```python
from build123d import *

# Parameters (mm, degrees)
F0_R     = 15
F1_DEPTH = 120
F2_W     = 20
F2_H     = 20
F3_DEPTH = 31


with BuildPart() as f1:
    # F0 (on Front) → F1 (new body)
    with BuildSketch(Plane.XZ):
        Circle(F0_R)
    extrude(amount=-F1_DEPTH)

    # F2 (on Right) → F3 (cut, symmetric)
    with BuildSketch(Plane.YZ):
        with Locations((20, 0)):
            Rectangle(F2_W, F2_H)
    extrude(amount=F3_DEPTH, both=True, mode=Mode.SUBTRACT)


solid = f1.part
```
CAD build for the part. Positions are in the model's coordinates, mm. A direction names the side the tool comes from. Round coordinates to 2 decimals unless told otherwise and drop trailing zeros. Loops run counter-clockwise (first coordinate to the right, second up) from the corner with the lowest first, then second, coordinate; pieces in that order, holes last. Notation, with made-up numbers: M 51.25,-8.5 L 70.25,-8.5 A19 cw 70.25,19.5 Z; hole C 19.25,-13 d3. An arc over 180 degrees is marked long. Use a Markdown table: item, result. Add a question column.
(1) Cut at C-C (z = -7). Give the cut face in (x, y), and give its area (3 significant figures).
(2) Which spindle directions (+Z, -Z, +X, -X, +Y, -Y) get a long thin tool onto all of the face, cutting with end or side? Do faces 1 (the face through (0, 120, 0)), 2 (the face through (0, 20, 10)). Say none if no direction does.
(3) Drill centre lines: line 1 (Y direction, x = -3, z = -9.5); line 2 (Z direction, x = 1.5, y = 75); line 3 (Z direction, x = -7, y = 85.5). Where is each one in solid material? Low to high.
(4) Cut at A-A (x = 0). Give the cut face in (y, z), and give its area (3 significant figures).
(5) Cut at B-B (z = 0). Give the cut face in (x, y).
(6) Flat gauge pins, fed straight in: pin 1 (1.5 mm diameter, centred on y = 86.5, z = 8, fed in from +X); pin 2 (4 mm diameter, centred on x = 4, y = 73, fed in from -Z); pin 3 (2 mm diameter, centred on y = 80.5, z = -3, fed in from +X). Where does each tip first touch, or does it go through?
(7) Cut at D-D (x = -8.75). Give the cut face in (y, z).
Geometry says:
| question | item | result |
|---|---|---|
| 1 | outline | M -13.27,0 L 13.27,0 L 13.27,10 L -13.27,10 Z; M -13.27,30 L 13.27,30 L 13.27,120 L -13.27,120 Z |
| 1 | area | 2,650 mm² |
| 2 | face 1 | +Z, -Z, +X, -X, +Y |
| 2 | face 2 | +X, -X |
| 3 | line 1 | y = 0 to 10, 30 to 120 |
| 3 | line 2 | z = -14.92 to 14.92 |
| 3 | line 3 | z = -13.27 to 13.27 |
| 4 | outline | M 0,-15 L 120,-15 L 120,15 L 0,15 Z; hole M 10,-10 L 30,-10 L 30,10 L 10,10 Z |
| 4 | area | 3,200 mm² |
| 5 | outline | M -15,0 L 15,0 L 15,10 L -15,10 Z; M -15,30 L 15,30 L 15,120 L -15,120 Z |
| 6 | pin 1 | stops at x = 13.13 |
| 6 | pin 2 | stops at z = -14.87 |
| 6 | pin 3 | stops at x = 14.87 |
| 7 | outline | M 0,-12.18 L 120,-12.18 L 120,12.18 L 0,12.18 Z; hole M 10,-10 L 30,-10 L 30,10 L 10,10 Z |
